The model under review builds one solid part; all positions refer to its coordinate system, in mm. A direction names the side the tool comes from. Coordinates: 2 decimals unless noted, no trailing zeros. Loops run counter-clockwise (first coordinate to the right, second up) from the corner with the lowest first, then second, coordinate; pieces in that order, holes last. Notation, with made-up numbers: (17, -3) - (34, -3) arc R19 ccw to (34, 21) - close; hole circle Ø7 at (10, 20). An arc over 180 degrees is marked (long way). Use a Markdown table: item, result. Add a question column.
1) For faces 1 (the cylindrical face through (-0.867, -3.905, 4.93)), 2 (the cylindrical face through (-6, 0, 92)), 3 (the cylindrical face through (-0.54, -17.44, 83.43)), list the 3-axis set-ups (+Z, -Z, +X, -X, +Y, -Y) from which the entire face can be reached by the end or side of a thin tool; tool diameter is ignored.
2) Add section C-C, the plane z = 32.5. Give the boundary of the cut face in (x, y).
3) To check wall thickness, follow L1, parallel to Y at x = 0, z = 83; L2, parallel to Z at x = -7, y = 15; L3, parallel to Z at x = -4, y = -4. State the ranges of each line that lie inside material, in increasing order. Write a range as [from, to].
4) Clearance check with flat-ended pins moving along their axes: pin 1 (3 mm diameter, centred on x = -0.5, z = 50.5, fed in from +Y); pin 2 (4 mm diameter, centred on x = -15, y = 0, fed in from +Z); pin 3 (8 mm diameter, centred on x = -8, z = 64.5, fed in from +Y); pin 4 (6 mm diameter, centred on x = -16, y = 4.5, fed in from -Z). State where each tip first meets the part, or that it passes through.
5) The part is to be moulded in two halves that separate along Y. For faces 4 (the cylindrical face through (-17.5, 0.1, 83.4)), 5 (the flat face through (0, 0, 0)), 6 (the cylindrical face through (-4.336, -19.524, 83.429)), say which applies: pulls with the +Y half, pulls with the -Y half, needs draft (parallel to the pull), parting line crosses it, or undercut.
6) Add section A-A, the plane y = 0. Give the boundary of the cut face in (x, z), and give its area (3 significant figures).
7) Add section D-D, the plane x = -5. Give the boundary of the cut face in (y, z).
8) Add section B-B, the plane x = -15. Give the boundary of the cut face in (y, z), and give its area (3 significant figures).
```python
from build123d import *

# Parameters (mm, degrees)
SKETCH1_R           = 6
BOSS_EXTRUDE1_DEPTH = 109.95
SKETCH2_R           = 20
SKETCH2_R_2         = 2.5
BOSS_EXTRUDE2_DEPTH = 3
SKETCH3_R           = 6
SKETCH3_R_2         = 4
CUT_EXTRUDE1_DEPTH  = 10


with BuildPart() as part:
    # Sketch1 → Boss-Extrude1 (new body)
    with BuildSketch(Plane.XY):
        Circle(SKETCH1_R)
    extrude(amount=BOSS_EXTRUDE1_DEPTH)

    # Sketch2 → Boss-Extrude2 (add)
    with BuildSketch(Plane.XY.offset(81.95)):
        Circle(SKETCH2_R)
        with Locations((0, 15)):
            Circle(SKETCH2_R_2, mode=Mode.SUBTRACT)
        with Locations((15, 0)):
            Circle(SKETCH2_R_2, mode=Mode.SUBTRACT)
        with Locations((0, -15)):
            Circle(SKETCH2_R_2, mode=Mode.SUBTRACT)
        with Locations((-15, 0)):
            Circle(SKETCH2_R_2, mode=Mode.SUBTRACT)
    extrude(amount=BOSS_EXTRUDE2_DEPTH)

    # Sketch3 → Cut-Extrude1 (cut)
    with BuildSketch(Plane.XY.offset(109.95)):
        Circle(SKETCH3_R)
        Circle(SKETCH3_R_2, mode=Mode.SUBTRACT)
    cut_extrude1 = extrude(amount=-CUT_EXTRUDE1_DEPTH, mode=Mode.SUBTRACT)

    # Mirror1: Cut-Extrude1 across plane
    add(cut_extrude1.mirror(Plane.XY.offset(54.975)), mode=Mode.SUBTRACT)


solid = part.part
```
From the geometry:
| question | item | result |
|---|---|---|
| 1 | face 1 | -Z |
| 1 | face 2 | +Z |
| 1 | face 3 | +Z, -Z |
| 2 | outline | circle Ø12 at (0, 0) |
| 3 | L1 | y = [-20, -17.5], [-12.5, 12.5], [17.5, 20] |
| 3 | L2 | z = [81.95, 84.95] |
| 3 | L3 | z = [10, 99.95] |
| 4 | pin 1 | stops at y = 6 |
| 4 | pin 2 | passes through |
| 4 | pin 3 | stops at y = 4.47 |
| 4 | pin 4 | stops at z = 81.95 |
| 5 | face 4 | undercut |
| 5 | face 5 | needs draft |
| 5 | face 6 | parting line crosses it |
| 6 | outline | (-20, 81.95) - (-17.5, 81.95) - (-17.5, 84.95) - (-20, 84.95) - close; (-12.5, 81.95) - (-6, 81.95) - (-6, 10) - (-4, 10) - (-4, 0) - (4, 0) - (4, 10) - (6, 10) - (6, 81.95) - (12.5, 81.95) - (12.5, 84.95) - (6, 84.95) - (6, 99.95) - (4, 99.95) - (4, 109.95) - (-4, 109.95) - (-4, 99.95) - (-6, 99.95) - (-6, 84.95) - (-12.5, 84.95) - close; (17.5, 81.95) - (20, 81.95) - (20, 84.95) - (17.5, 84.95) - close |
| 6 | area | 1,290 mm^2 |
| 7 | outline | (-19.36, 81.95) - (-3.32, 81.95) - (-3.32, 10) - (3.32, 10) - (3.32, 81.95) - (19.36, 81.95) - (19.36, 84.95) - (3.32, 84.95) - (3.32, 99.95) - (-3.32, 99.95) - (-3.32, 84.95) - (-19.36, 84.95) - close |
| 8 | outline | (-13.23, 81.95) - (-2.5, 81.95) - (-2.5, 84.95) - (-13.23, 84.95) - close; (2.5, 81.95) - (13.23, 81.95) - (13.23, 84.95) - (2.5, 84.95) - close |
| 8 | area | 64.4 mm^2 |
